Here's how the part is built. I have some questions about the finished solid (model axes, mm). A direction names the side the tool comes from. Round coordinates to 2 decimals unless told otherwise and drop trailing zeros. Loops run counter-clockwise (first coordinate to the right, second up) from the corner with the lowest first, then second, coordinate; pieces in that order, holes last. Notation, with made-up numbers: (29.5, -2) -> (83.5, -2) arc R22 ccw to (83.5, 28) -> close; hole circle Ø11 at (-3, -13). An arc over 180 degrees is marked (long way). One line per item, written item: value. Start each with the question number.
```python
from build123d import *

# Parameters (mm, degrees)
SKETCH_1_W          = 50
SKETCH_1_H          = 20
EXTRUDE_1_DEPTH     = 3
SKETCH_2_W          = 50
SKETCH_2_H          = 15
EXTRUDE_2_DEPTH     = 6
SKETCH_5_W          = 50
SKETCH_5_H          = 12
CUT_EXTRUDE_2_DEPTH = 3
SKETCH_4_R          = 1.65
SKETCH_4_R_2        = 0.5
SKETCH_4_R_3        = 0.75
CUT_EXTRUDE_1_DEPTH = 3


with BuildPart() as part:
    # 草图1 → 凸台-拉伸1 (new body)
    with BuildSketch(Plane.XY):
        Rectangle(SKETCH_1_W, SKETCH_1_H)
        with BuildLine():
            Line((-4.708438024, 2.5), (4.708438024, 2.5))
            ThreePointArc((4.708438024, 2.5), (5.261208823, 2.666666667), (5.629722688, 3.111111111))
            ThreePointArc((5.629722688, 3.111111111), (21, 0), (5.629722688, -3.111111111))
            ThreePointArc((5.629722688, -3.111111111), (5.261208823, -2.666666667), (4.708438024, -2.5))
            Line((4.708438024, -2.5), (-4.708438024, -2.5))
            ThreePointArc((-4.708438024, -2.5), (-5.261208823, -2.666666667), (-5.629722688, -3.111111111))
            ThreePointArc((-5.629722688, -3.111111111), (-21, 0), (-5.629722688, 3.111111111))
            ThreePointArc((-5.629722688, 3.111111111), (-5.261208823, 2.666666667), (-4.708438024, 2.5))
        make_face(mode=Mode.SUBTRACT)
        with BuildLine():
            Line((3.25, 5.5), (-3.25, 5.5))
            ThreePointArc((-3.25, 5.5), (-5, 7.25), (-3.25, 9))
            Line((-3.25, 9), (3.25, 9))
            ThreePointArc((3.25, 9), (5, 7.25), (3.25, 5.5))
        make_face(mode=Mode.SUBTRACT)
    extrude(amount=EXTRUDE_1_DEPTH)

    # 草图2 → 凸台-拉伸2 (add)
    with BuildSketch(Plane(origin=(0, 10, 0), x_dir=(1, 0, 0), z_dir=(0, 1, 0))):
        with Locations((0, -7.5)):
            Rectangle(SKETCH_2_W, SKETCH_2_H)
    extrude(amount=EXTRUDE_2_DEPTH)

    # 草图5 → 切除-拉伸2 (cut)
    with BuildSketch(Plane.XZ.offset(-10)):
        with Locations((0, 9)):
            Rectangle(SKETCH_5_W, SKETCH_5_H)
    extrude(amount=-CUT_EXTRUDE_2_DEPTH, mode=Mode.SUBTRACT)

    # 草图4 → 切除-拉伸1 (cut)
    with BuildSketch(Plane(origin=(0, 16, 0), x_dir=(1, 0, 0), z_dir=(0, 1, 0))):
        with Locations((0, -9)):
            Circle(SKETCH_4_R)
        with Locations((6.5, -9)):
            Circle(SKETCH_4_R_2)
        with Locations((-6.5, -9)):
            Circle(SKETCH_4_R_2)
        with Locations((11, -9)):
            Circle(SKETCH_4_R_3)
        with Locations((-10.5, -9)):
            Circle(SKETCH_4_R_3)
        with Locations((0, -4.5)):
            Circle(SKETCH_4_R_2)
        with Locations((0, -13.5)):
            Circle(SKETCH_4_R_2)
    extrude(amount=-CUT_EXTRUDE_1_DEPTH, mode=Mode.SUBTRACT)


solid = part.part
```
Q1. If I drill on line 1 along X through (y, z) = (14.6, 9); line 2 along Z through (x, y) = (-10.5, 14.4); line 3 along Z through (x, y) = (0, 14.15), over which ranges is the centre line in solid material (lowest first)?
Q2. Will these pins go through, and if not, where does the flat tip stop? P1, Ø3.5, axis at x = 9, z = 8, coming from the -Y side; P2, Ø1.2, axis at x = -10.5, z = 9, coming from the -Y side.
Q3. I want a section at B-B on z = 4.5. Please give me the cut outline in (x, y), plus the area to 3 significant figures.
Q4. If we mould it in two halves opening along X, with no side actions, what happens to faces 1 (the flat face through (0, 4, 3)), 2 (the flat face through (25, 5.8, 2.5)), 3 (the cylindrical face through (5.25, 2.66, 1.48))? For each: released by +X, released by -X, zero draft, split by the parting line, or undercut.
Q5. Which directions (+Z, -Z, +X, -X, +Y, -Y) give clear straight access to the entire face, cutting with the end or side of a thin tool? Please do faces 4 (the flat face through (0, 13, 6)), 5 (the cylindrical face through (-7, 15, 9)), 6 (the cylindrical face through (-5, 7.2, 1.5)).
Q6. I want a section at D-D on y = 5. Please give me the cut outline in (x, z) (3 decimals), plus the area to 3 significant figures.
Q7. I want a section at C-C on x = 0. Please give me the cut outline in (y, z).
Q8. I want a section at A-A on x = -13. Please give me the cut outline in (y, z).
Answers below:
1. line 1: x = -25 to -11.25, -9.75 to -7, -6 to -1.65, 1.65 to 6, 7 to 10.25, 11.75 to 25
1. line 2: z = 0 to 8.25, 9.75 to 15
1. line 3: z = 0 to 4, 5 to 7.35, 10.65 to 13, 14 to 15
2. P1: stops at y = 13
2. P2: passes through
3. outline: (-25, 13) -> (-0.5, 13) -> (-0.5, 16) -> (-25, 16) -> close; (0.5, 13) -> (25, 13) -> (25, 16) -> (0.5, 16) -> close
3. area: 147 mm^2
4. face 1: zero draft
4. face 2: released by +X
4. face 3: undercut
5. face 4: +Z, +X, -X, -Y
5. face 5: +Y, -Y
5. face 6: +Z, -Z
6. outline: (-25, 0) -> (-19.245, 0) -> (-19.245, 3) -> (-25, 3) -> close; (-6.755, 0) -> (6.755, 0) -> (6.755, 3) -> (-6.755, 3) -> close; (19.245, 0) -> (25, 0) -> (25, 3) -> (19.245, 3) -> close
6. area: 75.1 mm^2
7. outline: (-10, 0) -> (-2.5, 0) -> (-2.5, 3) -> (-10, 3) -> close; (2.5, 0) -> (5.5, 0) -> (5.5, 3) -> (2.5, 3) -> close; (9, 0) -> (16, 0) -> (16, 4) -> (13, 4) -> (13, 3) -> (9, 3) -> close; (13, 5) -> (16, 5) -> (16, 7.35) -> (13, 7.35) -> close; (13, 10.65) -> (16, 10.65) -> (16, 13) -> (13, 13) -> close; (13, 14) -> (16, 14) -> (16, 15) -> (13, 15) -> close
8. outline: (-10, 0) -> (-8, 0) -> (-8, 3) -> (-10, 3) -> close; (8, 0) -> (16, 0) -> (16, 15) -> (13, 15) -> (13, 3) -> (8, 3) -> close
